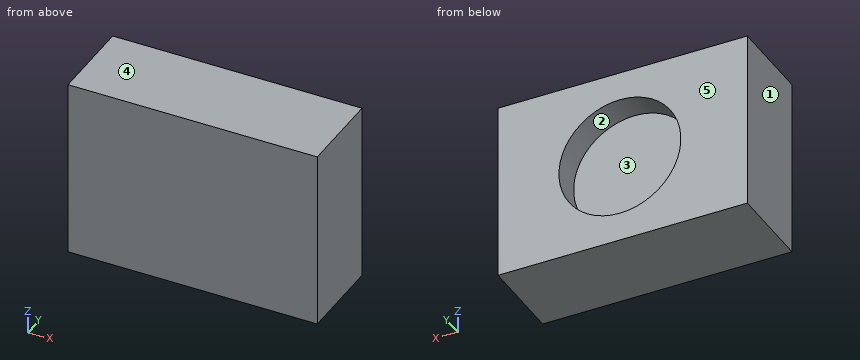
from build123d import *

# Parameters (mm, degrees)
CUT_EXTRUDE7_DEPTH               = 1010.950493836
CUT_EXTRUDE7_DEPTH_BACK          = 1010.950493836
SKETCH13_W                       = 48.176434887
SKETCH13_H                       = 155.804640487
SKETCH4_W                        = 600
SKETCH4_H                        = 44.158972604
CUT_EXTRUDE2_DEPTH               = 1010.950493836
SKETCH7_W                        = 159.807953253
SKETCH7_H                        = 69.49104999
BOSS_EXTRUDE7_DEPTH              = 5
FILLET5_R                        = 10
F_5_8_0_625_DIAMETER_HOLE1_D     = 15.875
F_5_8_0_625_DIAMETER_HOLE1_DEPTH = 30
F_5_8_0_625_DIAMETER_HOLE1_TIP   = 4.769331164
BOSS_EXTRUDE8_DEPTH              = 10
BOSS_EXTRUDE8_DEPTH_BACK         = 10
SKETCH16_W                       = 57.403477863
SKETCH16_H                       = 23.203595883
SKETCH17_W                       = 38.256761469
SKETCH17_H                       = 12.64819079
BOSS_EXTRUDE9_DEPTH              = 10
SKETCH18_W                       = 120
SKETCH18_H                       = 104.74536306
CUT_EXTRUDE8_DEPTH               = 161
FILLET6_R                        = 10
SKETCH19_R                       = 15
CUT_EXTRUDE9_DEPTH               = 7
CUT_EXTRUDE11_DEPTH              = 1010.950493856
CUT_EXTRUDE11_DEPTH_BACK         = 1010.950493856
SKETCH22_W                       = 1481.455902665
SKETCH22_H                       = 524.99926461
SKETCH22_W_2                     = 774.615564444
SKETCH22_H_2                     = 130
SKETCH23_W                       = 1033.221047575
SKETCH23_H                       = 313.410359552
SKETCH23_W_2                     = 790.959514037
SKETCH23_H_2                     = 163.499719248
CUT_EXTRUDE12_DEPTH              = 915.822387207
CUT_EXTRUDE13_DEPTH              = 908.868382599
CUT_EXTRUDE13_DEPTH_BACK         = 908.868382599
SKETCH24_W                       = 774.615564444
SKETCH24_H                       = 42.920513698
CUT_EXTRUDE14_DEPTH              = 908.868382607
CUT_EXTRUDE14_DEPTH_BACK         = 908.868382607
SKETCH25_W                       = 913.785959768
SKETCH25_H                       = 329.26502352
SKETCH25_W_2                     = 61.349903791
SKETCH25_H_2                     = 44.158972604


# Read off the part's stored shape, not the designer's step: Revolve1
with BuildPart() as part:
    # Revolve1 outline → Revolve1 (revolve)
    with BuildSketch(Plane.YX):
        with BuildLine():
            Line((0, 1000), (0, 0))
            ThreePointArc((0, 0), (70.710678154, 29.289321917), (100, 100.0000001))
            Line((100, 100.0000001), (100, 899.9999999))
            ThreePointArc((100, 899.9999999), (70.710678154, 970.710678083), (0, 1000))
        make_face()
    revolve(axis=Axis((0, 0, 0), (1, 0, 0)))

    # Sketch13 → Cut-Extrude7 (cut, two sides: drawn at the far end of the back side and taken through both)
    with BuildSketch(Plane(origin=(0, 0, 0), x_dir=(1, 0, 0), z_dir=(0, 1, 0)).offset(-CUT_EXTRUDE7_DEPTH_BACK)):
        with Locations((5.911782557, -3.075091589)):
            Rectangle(SKETCH13_W, SKETCH13_H)
    extrude(amount=CUT_EXTRUDE7_DEPTH + CUT_EXTRUDE7_DEPTH_BACK, mode=Mode.SUBTRACT)

    # Sketch4 → Cut-Extrude2 (cut, through all)
    with BuildSketch(Plane(origin=(0, 0, 0), x_dir=(1, 0, 0), z_dir=(0, 1, 0))):
        with Locations((595, 0)):
            Rectangle(SKETCH4_W, SKETCH4_H)
    extrude(amount=CUT_EXTRUDE2_DEPTH, mode=Mode.SUBTRACT)

    # Sketch7 → Boss-Extrude7 (add)
    with BuildSketch(Plane(origin=(0, 0, 0), x_dir=(1, 0, 0), z_dir=(0, 1, 0))):
        with Locations((745.885521462, -1.405844332)):
            Rectangle(SKETCH7_W, SKETCH7_H)
    extrude(amount=-BOSS_EXTRUDE7_DEPTH)

    # Fillet5
    fillet5_edges = [part.edges().sort_by_distance(p)[0] for p in [
        (30, -71.414284286, 0),
    ]]
    fillet(fillet5_edges, radius=FILLET5_R)

    # 5/8 (0.625) Diameter Hole1
    with Locations(Plane.ZY.offset(-30)):
        with Locations((0, 0)):
            Hole(F_5_8_0_625_DIAMETER_HOLE1_D / 2, depth=F_5_8_0_625_DIAMETER_HOLE1_DEPTH)
            with Locations((0, 0, -(F_5_8_0_625_DIAMETER_HOLE1_DEPTH + F_5_8_0_625_DIAMETER_HOLE1_TIP / 2))):  # 118° drill point
                Cone(0, F_5_8_0_625_DIAMETER_HOLE1_D / 2, F_5_8_0_625_DIAMETER_HOLE1_TIP, mode=Mode.SUBTRACT)

    # Sketch16 → Boss-Extrude8 (add, two sides: drawn at the far end of the back side and taken through both)
    with BuildSketch(Plane.XY.offset(-BOSS_EXTRUDE8_DEPTH_BACK)):
        with Locations((738.294537666, -11.601797942)):
            Rectangle(SKETCH16_W, SKETCH16_H)
    extrude(amount=BOSS_EXTRUDE8_DEPTH + BOSS_EXTRUDE8_DEPTH_BACK)

    # Sketch17 → Boss-Extrude9 (add)
    with BuildSketch(Plane.XY.offset(-22.079486302)):
        with Locations((787.071835847, 6.324095395)):
            Rectangle(SKETCH17_W, SKETCH17_H)
    extrude(amount=-BOSS_EXTRUDE9_DEPTH)

    # Sketch18 → Cut-Extrude8 (cut)
    with BuildSketch(Plane(origin=(0, 0, 0), x_dir=(1, 0, 0), z_dir=(0, 1, 0))):
        with Locations((204.992275313, 0)):
            Rectangle(SKETCH18_W, SKETCH18_H)
    extrude(amount=CUT_EXTRUDE8_DEPTH, mode=Mode.SUBTRACT)

    # Fillet6
    fillet6_edges = [part.edges().sort_by_distance(p)[0] for p in [
        (144.992275313, 42.594313674, -52.37268153),
        (144.992275313, 42.594313674, 52.37268153),
        (264.992275313, 42.594313674, 52.37268153),
        (264.992275313, 42.594313674, -52.37268153),
    ]]
    fillet(fillet6_edges, radius=FILLET6_R)

    # Sketch19 → Cut-Extrude9 (cut)
    with BuildSketch(Plane(origin=(0, 0, 0), x_dir=(1, 0, 0), z_dir=(0, 1, 0))):
        with Locations(Location((865, 0, 0), (0, 0, 270))):
            Circle(SKETCH19_R)
    extrude(amount=-CUT_EXTRUDE9_DEPTH, mode=Mode.SUBTRACT)

    # Sketch22 → Cut-Extrude11 (cut, two sides: drawn at the far end of the back side and taken through both)
    with BuildSketch(Plane(origin=(0, 0, 0), x_dir=(1, 0, 0), z_dir=(0, 1, 0)).offset(-CUT_EXTRUDE11_DEPTH_BACK)):
        with Locations((406.155110175, 0)):
            Rectangle(SKETCH22_W, SKETCH22_H)
        with Locations((512.692217778, 0)):
            Rectangle(SKETCH22_W_2, SKETCH22_H_2, mode=Mode.SUBTRACT)
    extrude(amount=CUT_EXTRUDE11_DEPTH + CUT_EXTRUDE11_DEPTH_BACK, mode=Mode.SUBTRACT)

    # Sketch23 → Cut-Extrude12 (cut, through all)
    with BuildSketch(Plane.XY.offset(65)):
        with Locations((481.89787613, -1.932796335)):
            Rectangle(SKETCH23_W, SKETCH23_H)
        with Locations((520.864192575, 60.415600646)):
            Rectangle(SKETCH23_W_2, SKETCH23_H_2, mode=Mode.SUBTRACT)
    extrude(amount=-CUT_EXTRUDE12_DEPTH, mode=Mode.SUBTRACT)

    # Sketch24 → Cut-Extrude13 (cut, two sides: drawn at the far end of the back side and taken through both)
    with BuildSketch(Plane(origin=(0, 0, 0), x_dir=(1, 0, 0), z_dir=(0, 1, 0)).offset(-CUT_EXTRUDE13_DEPTH_BACK)):
        with Locations((512.692217778, -43.539743151)):
            Rectangle(SKETCH24_W, SKETCH24_H)
    extrude(amount=CUT_EXTRUDE13_DEPTH + CUT_EXTRUDE13_DEPTH_BACK, mode=Mode.SUBTRACT)

    # Sketch25 → Cut-Extrude14 (cut, two sides: drawn at the far end of the back side and taken through both)
    with BuildSketch(Plane(origin=(0, 0, 0), x_dir=(1, 0, 0), z_dir=(0, 1, 0)).offset(-CUT_EXTRUDE14_DEPTH_BACK)):
        with Locations((557.248723254, -2.517184657)):
            Rectangle(SKETCH25_W, SKETCH25_H)
        with Locations((864.325048104, 0)):
            Rectangle(SKETCH25_W_2, SKETCH25_H_2, mode=Mode.SUBTRACT)
    extrude(amount=CUT_EXTRUDE14_DEPTH + CUT_EXTRUDE14_DEPTH_BACK, mode=Mode.SUBTRACT)


solid = part.part
Geometry check sheet. Reference: the model listing, model coordinates, mm. Face numbers are marked on the shaded views. A direction names the side the tool comes from. Coordinates: 2 decimals unless noted, no trailing zeros. Loops run counter-clockwise (first coordinate to the right, second up) from the corner with the lowest first, then second, coordinate; pieces in that order, holes last. Notation, with made-up numbers: (63.25, 27.5) - (89.25, 27.5) arc R10 cw to (89.25, 41.5) - close; hole circle Ø3 at (30, -27.5). An arc over 180 degrees is marked (long way). Use one line per item in the form item = value. Start each with the question number.
Item 1: Mould release check, pull along Z, two halves, no side actions. Record for the marked faces 3, 4 and 5: +Z half, -Z half, draft (parallel to the pull), parting line (faces both ways), or undercut.
Item 2: Tool access check on the marked faces 1 and 2. Record the directions out of +Z, -Z, +X, -X, +Y, -Y that give a thin tool (end or side, any length) a straight path to the whole face; none if there is none.
Item 3: Gauge pin test, flat end, axial feed: pin 1 (18 mm diameter, centred on x = 865, z = 0, fed in from +Y). Record the tip position at first contact, or that the pin passes through.
Item 4: Section check A-A, the plane x = 865. Enter the section's corners in (y, z).
Item 5: Thickness scan on probe 1 along X at (y, z) = (-5, 0); probe 2 along Y at (x, z) = (875, 10.5); probe 3 along X at (y, z) = (-1.75, -13). Record the ranges inside material, lowest first.
Item 6: Section check B-B, the plane z = 0. Enter the section's corners in (x, y), and give its area (3 significant figures).
Computed:
q1.face_3 = undercut
q1.face_4 = +Z half
q1.face_5 = draft
q2.face_1 = +Z, -Z, -X, +Y, -Y
q2.face_2 = +Y
q3.pin_1 = -7
q4.outline = (-21.33, -22.08) - (0, -22.08) - (0, -15) - (-7, -15) - (-7, 15) - (0, 15) - (0, 22.08) - (-21.33, 22.08) - close
q5.probe_1 = 833.65 to 850, 880 to 895
q5.probe_2 = -21.33 to -7
q5.probe_3 = 833.65 to 857.52, 872.48 to 895
q6.outline = (833.65, -21.33) - (895, -21.33) - (895, 0) - (880, 0) - (880, -7) - (850, -7) - (850, 0) - (833.65, 0) - close
q6.area = 1,100 mm2
